Read the model definition and answer for the solid it produces. Units are mm, in the model's axes. Face numbers are marked on the shaded views. Coordinates: 2 decimals unless noted, no trailing zeros. Write each loop counter-clockwise with the first axis right and the second up, starting at its lowest first coordinate (ties: lowest second). Pieces come first, ordered by that corner, then holes.
(1) The part is cut by section B-B, the plane y = 2.75. Determine the outline of the cut face in (x, z).
(2) The part is cut by section C-C, the plane z = -5. Determine the outline of the cut face in (x, y), and give its area (3 significant figures).
(3) The part is cut by section D-D, the plane x = 3. Determine the outline of the cut face in (y, z), and give its area (3 significant figures).
(4) The part is cut by section A-A, the plane z = -17. Determine the outline of the cut face in (x, y), and give its area (3 significant figures).
(5) Straight lines are drawn through the part: line 1 along Z through (x, y) = (17.5, -2); line 2 along Y through (x, z) = (16.5, -17.5); line 3 along X through (y, z) = (1.8, -5). For each, find the intervals that lie inside material, in ascending order.
(6) Given pin 1 (12.5 mm diameter, centred on x = 26.5, z = -9, fed in from -Y); pin 2 (6 mm diameter, centred on y = 1, z = -16, fed in from +X); pin 3 (3.5 mm diameter, centred on x = 3, z = -5, fed in from +Y); pin 4 (2.5 mm diameter, centred on y = 5.5, z = -23, fed in from -X), each flat-ended and moving along its own axis, determine where each tip first touches the part or whether it passes through.
(7) Determine the mould class of the marked faces 1, 2 and 3 for opening direction Z: pulls with the +Z half, pulls with the -Z half, needs draft (parallel to the pull), parting line crosses it, or undercut.
```python
from build123d import *

# Parameters (mm, degrees)
BOSS_EXTRU_1_DEPTH      = 4
ESQUISSE2_R             = 2
ENL_V_MAT_EXTRU_1_DEPTH = 4
ESQUISSE4_W             = 35
ESQUISSE4_H             = 10
BOSS_EXTRU_2_DEPTH      = 4


with BuildPart() as part:
    # Esquisse1 → Boss.-Extru.1 (new body)
    with BuildSketch(Plane(origin=(0, 0, 0), x_dir=(1, 0, 0), z_dir=(0, 1, 0))):
        Polygon((0, 0), (45, 25), (0, 25), align=None)
    extrude(amount=BOSS_EXTRU_1_DEPTH)

    # Esquisse2 → Enlèv. mat.-Extru.1 (cut)
    with BuildSketch(Plane(origin=(0, 4, 0), x_dir=(1, 0, 0), z_dir=(0, 1, 0))):
        with Locations(Location((3, 17, 0), (0, 0, 270))):
            Circle(ESQUISSE2_R)
        with Locations(Location((3, 5, 0), (0, 0, 270))):
            Circle(ESQUISSE2_R)
    extrude(amount=-ENL_V_MAT_EXTRU_1_DEPTH, mode=Mode.SUBTRACT)

    # Esquisse4 → Boss.-Extru.2 (add)
    with BuildSketch(Plane(origin=(0, 0, -25), x_dir=(-1, 0, 0), z_dir=(0, 0, -1))):
        with Locations((-27.5, 2)):
            Rectangle(ESQUISSE4_W, ESQUISSE4_H)
    extrude(amount=-BOSS_EXTRU_2_DEPTH)


solid = part.part
```
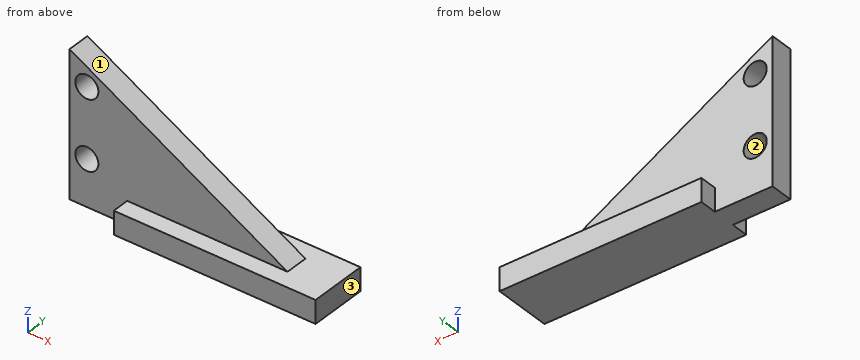
Computed:
1. outline: (0, -25) - (45, -25) - (45, -21) - (37.8, -21) - (0, 0) - close; hole circle Ø4 at (3, -17); hole circle Ø4 at (3, -5)
2. outline: (0, 0) - (1, 0) - (1, 4) - (0, 4) - close; (5, 0) - (9, 0) - (9, 4) - (5, 4) - close
2. area: 20.0 mm2
3. outline: (0, -25) - (4, -25) - (4, -19) - (0, -19) - close; (0, -15) - (4, -15) - (4, -7) - (0, -7) - close; (0, -3) - (4, -3) - (4, -1.67) - (0, -1.67) - close
3. area: 61.3 mm2
4. outline: (0, 0) - (1, 0) - (1, 4) - (0, 4) - close; (5, 0) - (30.6, 0) - (30.6, 4) - (5, 4) - close
4. area: 106 mm2
5. line 1: z = -25 to -21
5. line 2: y = 0 to 4
5. line 3: x = 0 to 1, 5 to 9
6. pin 1: stops at y = 0
6. pin 2: stops at x = 34.2
6. pin 3: passes through
6. pin 4: stops at x = 10
7. face 1: pulls with the +Z half
7. face 2: undercut
7. face 3: needs draft
